Can you work these out from the model? Positions are in its coordinate system, mm. A direction names the side the tool comes from. Coordinates: 2 decimals unless noted, no trailing zeros. Order: outer loops, then holes, each group sorted by start corner. A loop starts at its lowest first (then second) coordinate and runs counter-clockwise, first axis right, second up. Notation, with made-up numbers: (34.25, -32) -> (64.25, -32) arc R17 cw to (64.25, -12) -> close; hole circle Ø8 at (4.25, 38). An arc over 180 degrees is marked (long way). Return JSON: item names as keys, results as strings. Group by question number.
1) If I drill on probe 1 along Y at (x, z) = (53.5, 3.75); probe 2 along X at (y, z) = (1.8, 5.5), over which ranges is the centre line in solid material (lowest first)? Write a range as from..to.
2) For pin 1 (0.5 mm diameter, centred on y = 2, z = 4, fed in from -X); pin 2 (4.5 mm diameter, centred on x = 46.5, z = 6.5, fed in from +Y), each with a flat end and sliding along its axis, tell me the tip position at first contact or that it passes through.
3) For faces 1 (the flat face through (48, 1.143, 4)), 2 (the flat face through (38.354, 0.6, 4.4)), which set-ups out of +Z, -Z, +X, -X, +Y, -Y let a thin tool reach every point of the face, with its end or its side?
4) If we section it at A-A, the plane z = 2.5: Please give me the cut outline in (x, y), then the cut area to 3 significant figures.
5) If we section it at C-C, the plane y = 2.15: Please give me the cut outline in (x, z).
6) If we section it at B-B, the plane x = 41: Please give me the cut outline in (y, z).
Autodesk Inventor part; units mm, degrees
ref_plane "YZ Plane" through (0, 0, 0) normal (1, 0, 0) x (0, 1, 0)
ref_plane "XZ Plane" through (0, 0, 0) normal (0, 1, 0) x (-1, 0, 0)
ref_plane "XY Plane" through (0, 0, 0) normal (0, 0, 1) x (1, 0, 0)
sketch "Sketch1" plane through (0, 0, 0) normal (0, 0, 1) x (1, 0, 0)
  line L0 (38.354, 0) -> (76.2, 0)
  line L1 (76.2, 0) -> (76.2, 2.794)
  line L2 (76.2, 2.794) -> (57.15, 2.794)
  line L3 (57.15, 1.143) -> (57.15, 2.794)
  line L4 (38.354, 1.143) -> (57.15, 1.143)
  line L5 (38.354, 1.143) -> (38.354, 0)
  point P0 (0, 0)
extrude "Extrusion1" add sketch "Sketch1" along normal blind 8.89
properties part number "Mesh Test"
Result sheet:
{
 "1": {"probe 1": "y = 0..1.14", "probe 2": "x = 57.15..76.2"},
 "2": {"pin 1": "stops at x = 57.15", "pin 2": "stops at y = 1.14"},
 "3": {"face 1": "+Z, -Z, -X, +Y", "face 2": "+Z, -Z, -X, +Y, -Y"},
 "4": {"outline": "(38.35, 0) -> (76.2, 0) -> (76.2, 2.79) -> (57.15, 2.79) -> (57.15, 1.14) -> (38.35, 1.14) -> close", "area": "74.7 mm2"},
 "5": {"outline": "(57.15, 0) -> (76.2, 0) -> (76.2, 8.89) -> (57.15, 8.89) -> close"},
 "6": {"outline": "(0, 0) -> (1.14, 0) -> (1.14, 8.89) -> (0, 8.89) -> close"}
}
